Part model, mm, in its own coordinate system. Round coordinates to 2 decimals unless told otherwise and drop trailing zeros. Write each loop counter-clockwise with the first axis right and the second up, starting at its lowest first coordinate (ties: lowest second). Pieces come first, ordered by that corner, then holes. Notation, with made-up numbers: (47.25, 41.25) -> (85.25, 41.25) arc R9 cw to (85.25, 47.25) -> close; hole circle Ø6 at (27, -12). An arc over 180 degrees is marked (long way). Use CSV: the item, a comma, the result in double quotes. Start each with the question number.
(1) Probe line 1 (X direction, y = 1.25, z = 30); line 2 (Y direction, x = -29.5, z = -2). List the from-to ranges inside material, lowest first. Write a range as [from, to].
(2) Saw through at A-A (y = 4.75). Give the cut face in (x, z), plus the area to 3 significant figures.
(3) Drop flat-ended pins along their axis: pin 1 (2 mm diameter, centred on y = 2.5, z = -32.5, fed in from -X); pin 2 (4 mm diameter, centred on x = -40, y = 5.5, fed in from -Z); pin 3 (6 mm diameter, centred on x = 31.82, z = 31.82, fed in from +Y). Give the stop position or say it passes through.
(4) Saw through at B-B (x = 48.5). Give the cut face in (y, z), plus the area to 3 significant figures.
(5) Saw through at C-C (z = 5.5). Give the cut face in (x, y), plus the area to 3 significant figures.
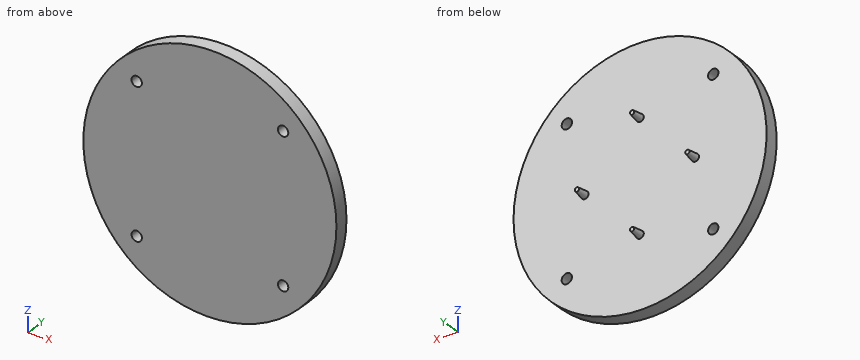
```python
from build123d import *

# Parameters (mm, degrees)
SKETCH1_R            = 55
BOSS_EXTRUDE1_DEPTH  = 6.35
SKETCH2_R            = 1.625
BOSS_EXTRUDE2_DEPTH  = 5
BOSS_EXTRUDE2_TAPER  = 8
M4_CLEARANCE_HOLE1_D = 4.5


with BuildPart() as part:
    # Sketch1 → Boss-Extrude1 (new body)
    with BuildSketch(Plane(origin=(0, 0, 0), x_dir=(1, 0, 0), z_dir=(0, 1, 0))):
        Circle(SKETCH1_R)
    extrude(amount=BOSS_EXTRUDE1_DEPTH)

    # Sketch2 → Boss-Extrude2 (add)
    with BuildSketch(Plane(origin=(0, 6.35, 0), x_dir=(1, 0, 0), z_dir=(0, 1, 0))):
        with Locations((0, -24)):
            Circle(SKETCH2_R)
        with Locations((-24, 0)):
            Circle(SKETCH2_R)
        with Locations((0, 24)):
            Circle(SKETCH2_R)
        with Locations((24, 0)):
            Circle(SKETCH2_R)
    extrude(amount=BOSS_EXTRUDE2_DEPTH, taper=BOSS_EXTRUDE2_TAPER)

    # M4 Clearance Hole1 (through all)
    with Locations(Plane(origin=(0, 6.35, 0), x_dir=(1, 0, 0), z_dir=(0, 1, 0))):
        with Locations((-31.819805153, 31.819805153), (31.819805153, 31.819805153), (31.819805153, -31.819805153), (-31.819805153, -31.819805153)):
            Hole(M4_CLEARANCE_HOLE1_D / 2)


solid = part.part
```
Answers:
1,line 1,"x = [-46.1, -33.14], [-30.5, 30.5], [33.14, 46.1]"
1,line 2,"y = [0, 6.35]"
2,outline,"circle Ø110 at (0, 0); hole circle Ø4.5 at (-31.82, -31.82); hole circle Ø4.5 at (-31.82, 31.82); hole circle Ø4.5 at (31.82, -31.82); hole circle Ø4.5 at (31.82, 31.82)"
2,area,"9,440 mm²"
3,pin 1,"stops at x = -45.09"
3,pin 2,"stops at z = -39.76"
3,pin 3,"stops at y = 6.35"
4,outline,"(0, -25.94) -> (6.35, -25.94) -> (6.35, 25.94) -> (0, 25.94) -> close"
4,area,"329 mm²"
5,outline,"(-54.72, 0) -> (54.72, 0) -> (54.72, 6.35) -> (-54.72, 6.35) -> close"
5,area,"695 mm²"
